For this review, take the finished solid that the model builds, in its own axes (mm). Face numbers are marked on the shaded views. A direction names the side the tool comes from. Coordinates: 2 decimals unless noted, no trailing zeros. Loops run counter-clockwise (first coordinate to the right, second up) from the corner with the lowest first, then second, coordinate; pieces in that order, holes last. Notation, with made-up numbers: M 30,-15.5 L 49,-15.5 A4 cw 49,-9.5 Z; hole C 65.5,-5.75 d11. An arc over 180 degrees is marked long. Put each result on its own line as item: value.
```python
from build123d import *

# Parameters (mm, degrees)
SKETCH1_W             = 30
SKETCH1_H             = 66
SKETCH1_R             = 7.875
BOSS_EXTRUDE1_DEPTH   = 50
SKETCH2_W             = 80
SKETCH2_H             = 63
CUT_EXTRUDE1_DEPTH    = 79.797208072
BOSS_EXTRUDE2_DEPTH   = 100
SKETCH5_R             = 5
CUT_EXTRUDE2_DEPTH    = 130.077496102
M5X0_8_TAPPED_HOLE1_D = 4.2
FILLET1_R             = 10
SKETCH10_R            = 17.5
CUT_EXTRUDE3_DEPTH    = 134.719856416


with BuildPart() as part:
    # Sketch1 → Boss-Extrude1 (new, symmetric)
    with BuildSketch(Plane.XY):
        with Locations((0, -20)):
            Rectangle(SKETCH1_W, SKETCH1_H)
        Circle(SKETCH1_R, mode=Mode.SUBTRACT)
        with Locations((0, -40)):
            Circle(SKETCH1_R, mode=Mode.SUBTRACT)
    extrude(amount=BOSS_EXTRUDE1_DEPTH, both=True)

    # Sketch2 → Cut-Extrude1 (cut, through all)
    with BuildSketch(Plane(origin=(15, 0, 0), x_dir=(0, 0, -1), z_dir=(1, 0, 0))):
        with Locations((0, -21.5)):
            Rectangle(SKETCH2_W, SKETCH2_H)
    extrude(amount=-CUT_EXTRUDE1_DEPTH, mode=Mode.SUBTRACT)

    # Sketch4 → Boss-Extrude2 (add)
    with BuildSketch(Plane.XY.offset(50)):
        Polygon((15, 13), (30.005154776, -43), (105, -43), (105, -53), (15, -53), align=None)
    extrude(amount=-BOSS_EXTRUDE2_DEPTH)

    # Sketch5 → Cut-Extrude2 (cut, through all)
    with BuildSketch(Plane(origin=(0, -43, 0), x_dir=(1, 0, 0), z_dir=(0, 1, 0))):
        with Locations(Location((66.5, 0, 0), (0, 0, 270))):
            Circle(SKETCH5_R)
    extrude(amount=-CUT_EXTRUDE2_DEPTH, mode=Mode.SUBTRACT)

    # M5x0.8 Tapped Hole1 (through all)
    with Locations(Plane(origin=(0, -43, 0), x_dir=(1, 0, 0), z_dir=(0, 1, 0))):
        with Locations((80.642135624, 14.142135624), (80.642135624, -14.142135624), (52.357864376, 14.142135624), (52.357864376, -14.142135624)):
            Hole(M5X0_8_TAPPED_HOLE1_D / 2)

    # Fillet1
    fillet1_edges = [part.edges().sort_by_distance(p)[0] for p in [
        (15, 13, 0),
        (30.005154776, -43, 0),
        (105, -48, 50),
        (105, -48, -50),
        (-15, -53, -45),
        (-15, -53, 45),
        (15, 10, 0),
    ]]
    fillet(fillet1_edges, radius=FILLET1_R)

    # Sketch10 → Cut-Extrude3 (cut, through all)
    with BuildSketch(Plane(origin=(0, 13, 0), x_dir=(1, 0, 0), z_dir=(0, 1, 0))):
        with Locations(Location((26.5, 0, 0), (0, 0, 274.980086745))):
            Circle(SKETCH10_R)
    extrude(amount=-CUT_EXTRUDE3_DEPTH, mode=Mode.SUBTRACT)


solid = part.part
```
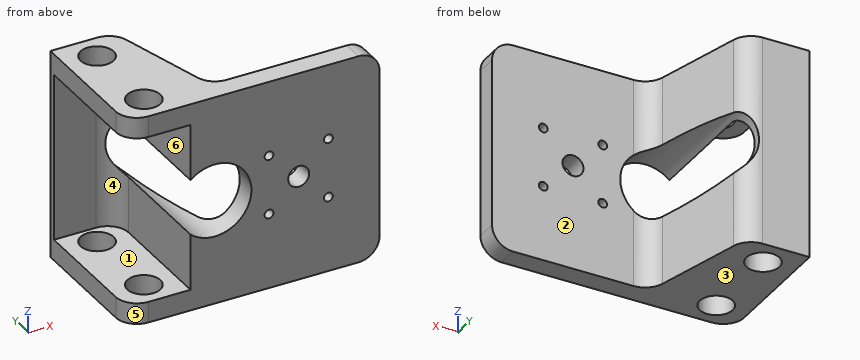
(1) For pin 1 (4 mm diameter, centred on x = -2, z = 31, fed in from -Y); pin 2 (1.5 mm diameter, centred on x = 45.5, z = -36, fed in from +Y); pin 3 (21.5 mm diameter, centred on y = -37, z = 21, fed in from -X), all flat-tipped, find the tip position at first contact; note any pin that passes through.
Determined:
pin 1: stops at y = 10
pin 2: stops at y = -43
pin 3: stops at x = 15
(2) Add section D-D (z = 33). Write out the cut boundary in (x, y), plus the area to 3 significant figures.
Determined:
outline: M -15,10 L 5,10 A10 cw 15,0 L 15,-53 L 105,-53 L 105,-43 L 37.68,-43 A10 cw 28.02,-35.59 L 16.99,5.59 A10 ccw 7.33,13 L -15,13 Z
area: 1,430 mm^2
(3) Add section B-B (z = 0.5). Write out the cut boundary in (x, y), plus the area to 3 significant figures.
Determined:
outline: M -15,10 L 5,10 A10 cw 9.01,9.16 L 9.01,12.86 A10 ccw 7.33,13 L -15,13 Z; M 43.99,-53 L 61.53,-53 L 61.53,-43 L 43.99,-43 Z; M 71.47,-53 L 105,-53 L 105,-43 L 71.47,-43 Z
area: 584 mm^2
(4) Add section A-A (x = 0). Write out the cut boundary in (y, z) (3 decimals).
Determined:
outline: M -53,-50 L -47.875,-50 L -47.875,-40 L -53,-40 Z; M -53,40 L -47.875,40 L -47.875,50 L -53,50 Z; M -32.125,-50 L -7.875,-50 L -7.875,-40 L -32.125,-40 Z; M -32.125,40 L -7.875,40 L -7.875,50 L -32.125,50 Z; M 7.875,-50 L 13,-50 L 13,50 L 7.875,50 L 7.875,40 L 10,40 L 10,-40 L 7.875,-40 Z
(5) Add section C-C (x = 19.5). Write out the cut boundary in (y, z).
Determined:
outline: M -53,-50 L -3.79,-50 L -3.79,-16.04 L -53,-16.04 Z; M -53,16.04 L -3.79,16.04 L -3.79,50 L -53,50 Z
(6) Draft analysis for pull direction Z (two halves, no side actions). For the marked faces 1, 2, 3 and 4, state which applies: +Z half, -Z half, draft (parallel to the pull), parting line (faces both ways), or undercut.
Determined:
face 1: undercut
face 2: draft
face 3: -Z half
face 4: undercut
(7) Wall thickness on line 1 along Y through (x, z) = (0, -45) (3 decimals); line 2 along Z through (x, y) = (11, -1); line 3 along Z through (x, y) = (54, -45.5): over which ranges is each line inside the solid? List them lowest first. Write a range as [from, to].
Determined:
line 1: y = [-53, -47.875], [-32.125, -7.875], [7.875, 13]
line 2: z = [-50, -40], [40, 50]
line 3: z = [-50, -15.45], [-12.83, 12.83], [15.45, 50]
(8) Tool access review of the marked faces 5 and 6: name each direction out of +Z, -Z, +X, -X, +Y, -Y from which nothing blocks a thin tool from reaching the whole face with its end or side.
Determined:
face 5: +Z, -Z, -X, -Y
face 6: -X, -Y
